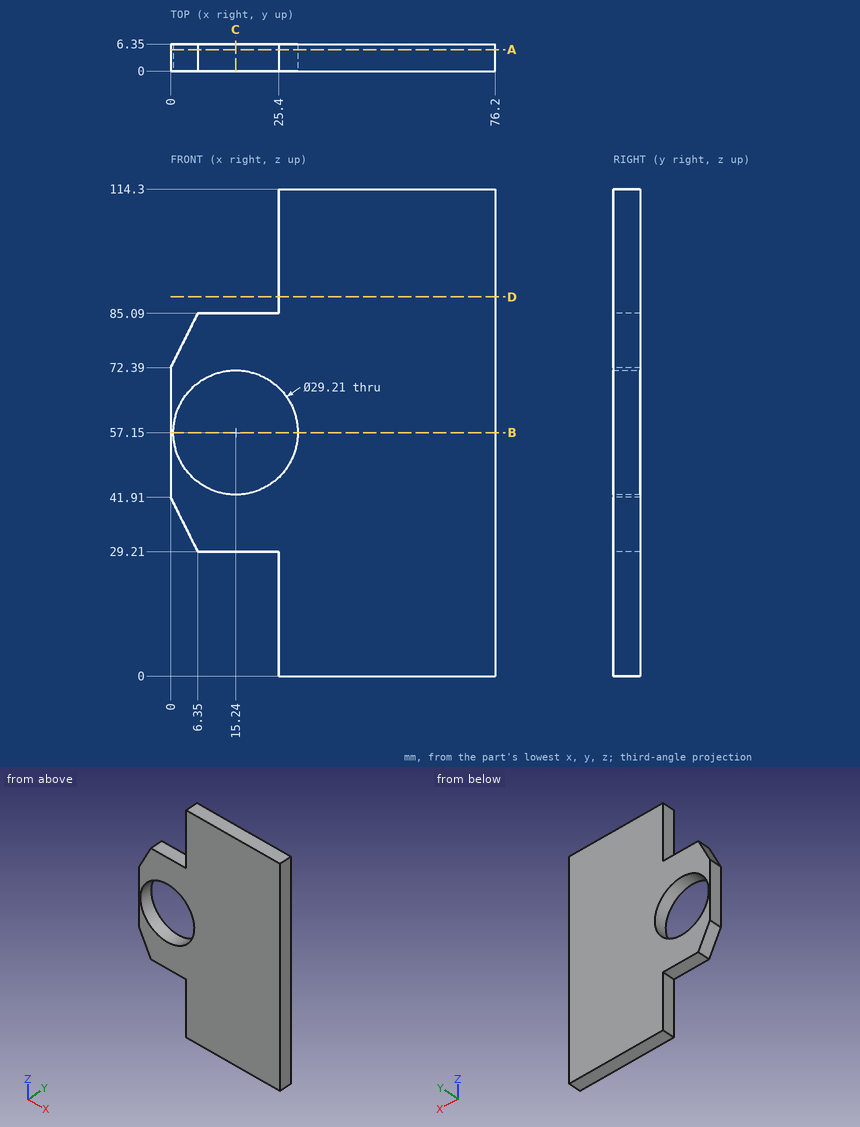
Could you check a few things on this drawing? It's one solid part, dimensions in mm from its lowest x, y, z. Coordinates: 2 decimals unless noted, no trailing zeros. Write each loop counter-clockwise with the first axis right and the second up, starting at its lowest first coordinate (ties: lowest second). Pieces come first, ordered by that corner, then holes.
1) If we section it at C-C (x = 15.24): List the corners of the cut face in (y, z) for me (3 decimals).
Filled in:
outline: (0, 29.21) - (6.35, 29.21) - (6.35, 42.545) - (0, 42.545) - close; (0, 71.755) - (6.35, 71.755) - (6.35, 85.09) - (0, 85.09) - close
2) I'm going to push flat-ended pins straight in: pin 1 (3 mm diameter, centred on y = 2, z = 93.5, fed in from -X); pin 2 (1 mm diameter, centred on x = 16, y = 4, fed in from -Z); pin 3 (1.9 mm diameter, centred on x = 18.5, y = 4.5, fed in from +Z). Where does each tip first touch, or does it pass through?
Filled in:
pin 1: stops at x = 25.4
pin 2: stops at z = 29.21
pin 3: stops at z = 85.09
3) If we section it at B-B (z = 57.15): List the corners of the cut face in (x, y) for me (3 decimals), plus the area to 3 significant figures.
Filled in:
outline: (0, 0) - (0.635, 0) - (0.635, 6.35) - (0, 6.35) - close; (29.845, 0) - (76.2, 0) - (76.2, 6.35) - (29.845, 6.35) - close
area: 298 mm2
4) If we section it at D-D (z = 89): List the corners of the cut face in (x, y) for me, plus the area to 3 significant figures.
Filled in:
outline: (25.4, 0) - (76.2, 0) - (76.2, 6.35) - (25.4, 6.35) - close
area: 323 mm2
5) If I drill on line 1 (X direction, y = 3.5, z = 57); line 2 (Z direction, x = 14.5, y = 3.75); line 3 (X direction, y = 0.75, z = 92.5), over which ranges is the centre line in solid material (lowest first)?
Filled in:
line 1: x = 0 to 0.64, 29.84 to 76.2
line 2: z = 29.21 to 42.56, 71.74 to 85.09
line 3: x = 25.4 to 76.2
6) If we section it at A-A (y = 5): List the corners of the cut face in (x, z) for me (3 decimals).
Filled in:
outline: (0, 41.91) - (6.35, 29.21) - (25.4, 29.21) - (25.4, 0) - (76.2, 0) - (76.2, 114.3) - (25.4, 114.3) - (25.4, 85.09) - (6.35, 85.09) - (0, 72.39) - close; hole circle Ø29.21 at (15.24, 57.15)
